The model under review builds one solid part; all positions refer to its coordinate system, in mm. Face numbers are marked on the shaded views. A direction names the side the tool comes from. Round coordinates to 2 decimals unless told otherwise and drop trailing zeros. Write each loop counter-clockwise with the first axis right and the second up, starting at its lowest first coordinate (ties: lowest second). Pieces come first, ordered by that corner, then holes. Notation, with made-up numbers: (54, -18.75) - (79, -18.75) arc R29 ccw to (79, 13.25) - close; hole circle Ø11 at (27.5, -18.75). An arc over 180 degrees is marked (long way). Write each question's results on one line, items separated by ' | '.
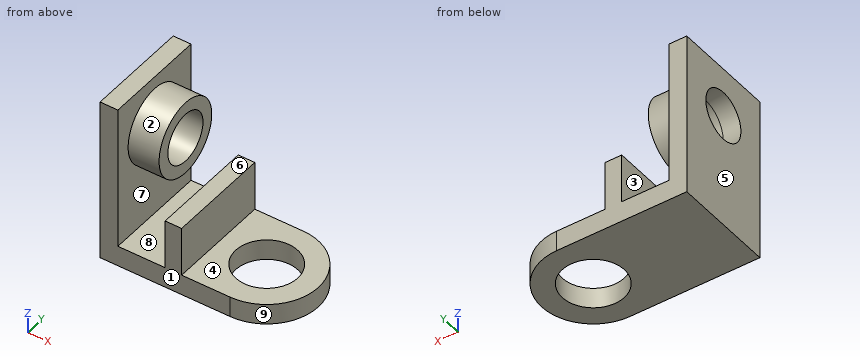
```python
from build123d import *

# Parameters (mm, degrees)
F1_DEPTH = 10
F2_W     = 8
F2_H     = 50
F3_DEPTH = 24
F4_W     = 8.6245508865
F4_H     = 50
F5_DEPTH = 70
F6_R     = 18
F6_R_2   = 12
F7_DEPTH = 15
F8_R     = 12
F9_DEPTH = 8.6245508865


with BuildPart() as f1:
    # F0 (on Top) → F1 (new body)
    with BuildSketch(Plane.XY):
        with BuildLine():
            Line((0, 50), (0, 0))
            Line((0, 0), (63, 0))
            ThreePointArc((63, 0), (88, 25), (63, 50))
            Line((63, 50), (0, 50))
        make_face()
        with BuildLine():
            ThreePointArc((78, 25), (52.3933982822, 14.3933982822), (63, 40))
            ThreePointArc((63, 40), (73.6066017178, 35.6066017178), (78, 25))
        make_face(mode=Mode.SUBTRACT)
    extrude(amount=F1_DEPTH)

    # F2 (on face) → F3 (join)
    with BuildSketch(Plane.XY.offset(10)):
        with Locations((35.5, 25)):
            Rectangle(F2_W, F2_H)
    extrude(amount=F3_DEPTH)

    # F4 (on face) → F5 (join)
    with BuildSketch(Plane.XY.offset(10)):
        with Locations((4.3122754432, 25)):
            Rectangle(F4_W, F4_H)
    extrude(amount=F5_DEPTH)

    # F6 (on face) → F7 (join)
    with BuildSketch(Plane.YZ.offset(8.6245508865)):
        with Locations((25, 56)):
            Circle(F6_R)
        with Locations((25, 56)):
            Circle(F6_R_2, mode=Mode.SUBTRACT)
    extrude(amount=F7_DEPTH)

    # F8 (on face) → F9 (cut, through all)
    with BuildSketch(Plane.YZ.offset(8.6245508865)):
        with Locations((25, 56)):
            Circle(F8_R)
    extrude(amount=-F9_DEPTH, mode=Mode.SUBTRACT)


solid = f1.part
```
Q1. For probe 1 along Z at (x, y) = (20, 25); probe 2 along X at (y, z) = (27, 13.5); probe 3 along Z at (x, y) = (6.75, 25), list the stretches that pass through material, from the lowest coordinate up.
Evaluation:
probe 1: z = 0 to 10, 38 to 44, 68 to 74 | probe 2: x = 0 to 8.62, 31.5 to 39.5 | probe 3: z = 0 to 44, 68 to 80
Q2. Insertion check: P1, Ø2.5, axis at x = 35, y = 13.5, coming from the +Z side; P2, Ø10, axis at x = 10.5, y = 43.5, coming from the +Z side; P3, Ø11, axis at y = 16.5, z = 55, coming from the +X side; P4, Ø11.5, axis at x = 18, y = 37.5, coming from the +Z side. Each pin has a flat end and moves straight along its axis. Give the tip position at first contact, or say it passes through.
Evaluation:
P1: stops at z = 34 | P2: stops at z = 80 | P3: stops at x = 23.62 | P4: stops at z = 72.69
Q3. We need section D-D (z = 20.5). State the section outline as (x, y) points.
Evaluation:
outline: (0, 0) - (8.62, 0) - (8.62, 50) - (0, 50) - close; (31.5, 0) - (39.5, 0) - (39.5, 50) - (31.5, 50) - close
Q4. We need section C-C (x = 16.5). State the section outline as (y, z) points.
Evaluation:
outline: (0, 0) - (50, 0) - (50, 10) - (0, 10) - close; circle Ø36 at (25, 56); hole circle Ø24 at (25, 56)
Q5. We need section A-A (y = 25). State the section outline as (x, z) points, plus the area to 3 significant figures.
Evaluation:
outline: (0, 0) - (48, 0) - (48, 10) - (39.5, 10) - (39.5, 34) - (31.5, 34) - (31.5, 10) - (8.62, 10) - (8.62, 38) - (23.62, 38) - (23.62, 44) - (0, 44) - close; (0, 68) - (23.62, 68) - (23.62, 74) - (8.62, 74) - (8.62, 80) - (0, 80) - close; (78, 0) - (88, 0) - (88, 10) - (78, 10) - close | area: 1,350 mm^2
Q6. The part is to be moulded in two halves that separate along X. For the marked faces 6, 7, 8 and 9, say which applies: released by +X, released by -X, zero draft, split by the parting line, or undercut.
Evaluation:
face 6: zero draft | face 7: undercut | face 8: undercut | face 9: released by +X
Q7. Tool access review of the marked faces 1, 2, 3, 4 and 5: name each direction out of +Z, -Z, +X, -X, +Y, -Y from which nothing blocks a thin tool from reaching the whole face with its end or side.
Evaluation:
face 1: +Z, -Z, +X, -X, -Y | face 2: +X | face 3: +Z, +Y, -Y | face 4: +Z, +X, +Y, -Y | face 5: +Z, -Z, -X, +Y, -Y
Q8. We need section B-B (z = 56). State the section outline as (x, y) points.
Evaluation:
outline: (0, 0) - (8.62, 0) - (8.62, 7) - (23.62, 7) - (23.62, 13) - (0, 13) - close; (0, 37) - (23.62, 37) - (23.62, 43) - (8.62, 43) - (8.62, 50) - (0, 50) - close
